Check sheet for the drawn part. Datum: minimum x, y, z corner. Units: mm. A direction names the side the tool comes from. Give positions to 0.01 mm unless a question says otherwise; leave off trailing zeros. Write each loop counter-clockwise with the first axis right and the second up, starting at its lowest first coordinate (ties: lowest second). Pieces come first, ordered by that corner, then holes. Notation, with made-up numbers: M 43.5,-28 L 70.5,-28 A15 ccw 70.5,-1 Z; hole C -17,39 d11. An arc over 180 degrees is marked long. Use CSV: the item, a comma, the result in double quotes. Start each with the question number.
1. Cross-section at D-D, the plane y = 55.5. Enter the section's corners in (x, z).
2. Cross-section at B-B, the plane y = 7. Enter the section's corners in (x, z) (3 decimals), and give its area (3 significant figures).
3. Cross-section at A-A, the plane x = 10. Enter the section's corners in (y, z).
4. Depth check by flat-ended pin: P1, Ø2.5, axis at y = 7, z = 11.475, coming from the +X side; P2, Ø19, axis at y = 34, z = 15, coming from the +X side; P3, Ø8, axis at x = 25.5, y = 12.5, coming from the +Z side; P4, Ø10, axis at y = 35, z = 34.5, coming from the -X side. Enter the tip coordinate at first touch or a pass-through.
5. Cross-section at C-C, the plane z = 27. Enter the section's corners in (x, y), and give its area (3 significant figures).
6. Scan lines: line 1 (Z direction, x = 54.05, y = 73) (3 decimals); line 2 (X direction, y = 70, z = 1.2); line 3 (Y direction, x = 10, z = 1.9). Record each from-to range of solid material in increasing order.
7. Access from +Z, -Z, +X, -X, +Y, -Y to the whole of each face (thin tool, end or side, straight path). Record for the marked faces 1, 2 and 3.
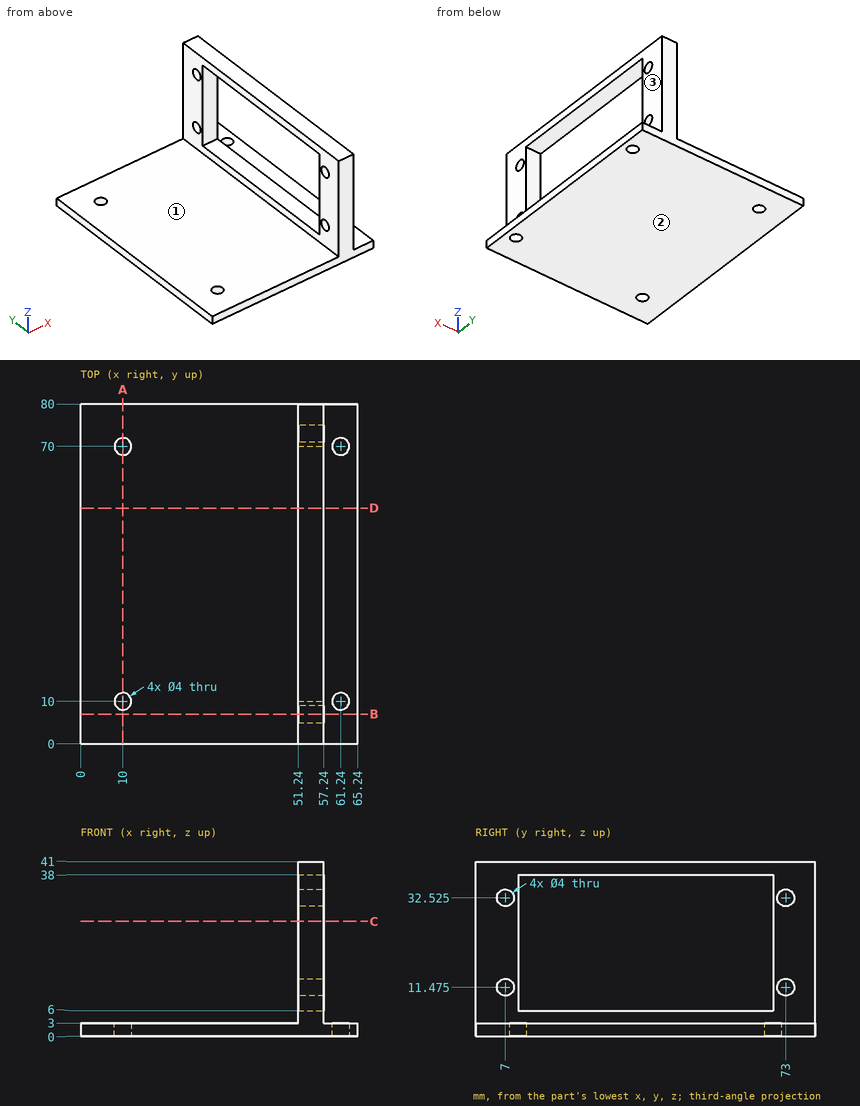
Worked answers:
1,outline,"M 0,0 L 65.24,0 L 65.24,3 L 57.24,3 L 57.24,6 L 51.24,6 L 51.24,3 L 0,3 Z; M 51.24,38 L 57.24,38 L 57.24,41 L 51.24,41 Z"
2,outline,"M 0,0 L 65.24,0 L 65.24,3 L 57.24,3 L 57.24,9.475 L 51.24,9.475 L 51.24,3 L 0,3 Z; M 51.24,13.475 L 57.24,13.475 L 57.24,30.525 L 51.24,30.525 Z; M 51.24,34.525 L 57.24,34.525 L 57.24,41 L 51.24,41 Z"
2,area,"376 mm^2"
3,outline,"M 0,0 L 8,0 L 8,3 L 0,3 Z; M 12,0 L 68,0 L 68,3 L 12,3 Z; M 72,0 L 80,0 L 80,3 L 72,3 Z"
4,P1,"passes through"
4,P2,"stops at x = 57.24"
4,P3,"stops at z = 3"
4,P4,"stops at x = 51.24"
5,outline,"M 51.24,0 L 57.24,0 L 57.24,10 L 51.24,10 Z; M 51.24,70 L 57.24,70 L 57.24,80 L 51.24,80 Z"
5,area,"120 mm^2"
6,line 1,"z = 0 to 9.475, 13.475 to 30.525, 34.525 to 41"
6,line 2,"x = 0 to 8, 12 to 59.24, 63.24 to 65.24"
6,line 3,"y = 0 to 8, 12 to 68, 72 to 80"
7,face 1,"+Z, -X, +Y, -Y"
7,face 2,"-Z, +X, -X, +Y, -Y"
7,face 3,"+Z, +X, +Y, -Y"
